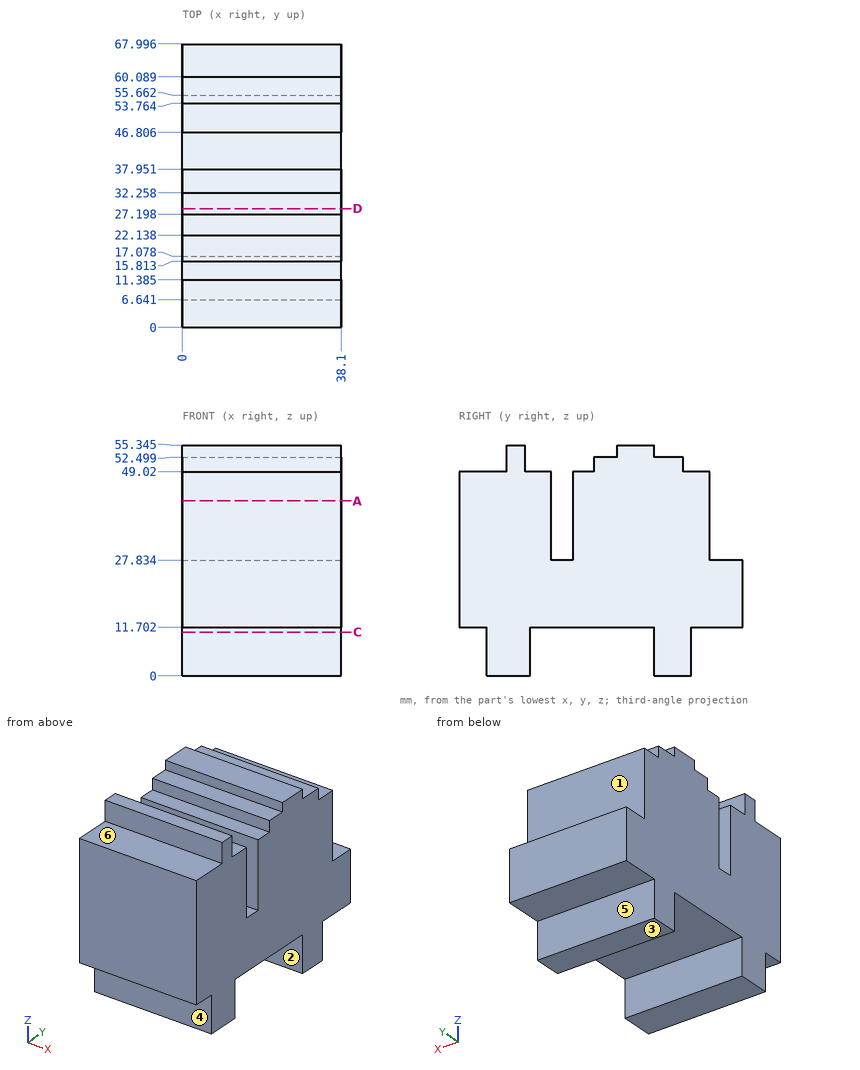
Source: three-view drawing plus pictorial views. Frame: mm from the lowest corner of the part. A direction names the side the tool comes from. Round coordinates to 2 decimals unless told otherwise and drop trailing zeros. Loops run counter-clockwise (first coordinate to the right, second up) from the corner with the lowest first, then second, coordinate; pieces in that order, holes last.
Q1. Mould query, pull axis Y, two halves, no side actions, for the marked faces 1, 2 and 3. Classes: pulls with the +Y half, pulls with the -Y half, needs draft (parallel to the pull), parting line crosses it, or undercut.
Q2. Section A-A, the plane z = 42. Return loops of the section in (x, y).
Q3. Ray query, line 1 (Y direction, x = 9, z = 29); line 2 (Y direction, x = 13, z = 7.5); line 3 (Z direction, x = 24.5, y = 38) (1 decimal). Return the intervals inside material, ascending.
Q4. First-contact query: P1, Ø12, axis at x = 34, z = 32, coming from the +Y side; P2, Ø4, axis at x = 26, y = 24.5, coming from the +Z side; P3, Ø4, axis at x = 12.5, z = 50.5, coming from the +Y side; P4, Ø6, axis at x = 17, z = 8.5, coming from the -Y side. Flat tips, straight axial feed; report the tip coordinate or a pass-through.
Q5. Section C-C, the plane z = 10.5. Return loops of the section in (x, y), plus the area to 3 significant figures.
Q6. Section D-D, the plane y = 28.5. Return loops of the section in (x, z), plus the area to 3 significant figures.
Q7. Access query for the marked faces 4, 5 and 6. Directions: +Z, -Z, +X, -X, +Y, -Y. A direction counts if a zero-diameter tool reaches every point of the face in a straight line with its end or side. Return the directions, or none.
Solutions:
1. face 1: pulls with the +Y half
1. face 2: undercut
1. face 3: needs draft
2. outline: (0, 0) - (38.1, 0) - (38.1, 22.14) - (0, 22.14) - close; (0, 27.2) - (38.1, 27.2) - (38.1, 60.09) - (0, 60.09) - close
3. line 1: y = 0 to 22.14, 27.2 to 60.09
3. line 2: y = 6.64 to 17.08, 46.81 to 55.66
3. line 3: z = 11.7 to 55.3
4. P1: stops at y = 68
4. P2: stops at z = 27.83
4. P3: stops at y = 60.09
4. P4: stops at y = 6.64
5. outline: (0, 6.64) - (38.1, 6.64) - (38.1, 17.08) - (0, 17.08) - close; (0, 46.81) - (38.1, 46.81) - (38.1, 55.66) - (0, 55.66) - close
5. area: 735 mm2
6. outline: (0, 11.7) - (38.1, 11.7) - (38.1, 49.02) - (0, 49.02) - close
6. area: 1,420 mm2
7. face 4: -Z, +X, -X, -Y
7. face 5: -Z, +X, -X, +Y
7. face 6: +Z, +X, -X, -Y
